Work out the finished part from the listing and answer in its coordinate system (mm). Round coordinates to 2 decimals unless told otherwise and drop trailing zeros. Loops run counter-clockwise (first coordinate to the right, second up) from the corner with the lowest first, then second, coordinate; pieces in that order, holes last. Notation, with made-up numbers: (-1.5, 32.25) - (48.5, 32.25) arc R17 ccw to (48.5, 55.25) - close; hole circle Ø7 at (55.5, 14.5). An arc over 180 degrees is marked (long way). Answer as CSV lines item,"result". Start each with the question number.
Q1. Straight lines are drawn through the part: L1, parallel to Y at x = 168.5, z = -34.5; L2, parallel to Y at x = -163, z = -490.5. For each, find the intervals that lie inside material, in ascending order. Write a range as [from, to].
Q2. Each of these flat-tipped pins is pushed along its axis until it touches: pin 1 Ø1.5 at (x, z) = (-8.5, -291) entering from -Y; pin 2 Ø4 at (x, y) = (173, -57.5) entering from -Z; pin 3 Ø4 at (x, y) = (180, -59) entering from +Z. Where does it stop, or does it pass through?
Q3. Section A-A on x = -110.5 is taken. Write down the section's boundary in (y, z).
Q4. Section B-B on z = -164 is taken. Write down the section's boundary in (x, y).
```python
from build123d import *

# Parameters (mm, degrees)
F0_W        = 457.2
F0_H        = 1828.8
F1_DEPTH    = 50.8
F2_W        = 25.4
F2_H        = 254
F3_DEPTH    = 25.4
F4_T1_DEPTH = 361.4104165052
F5_W        = 12.7
F5_H        = 57.15
F6_DEPTH    = 417.2741922717


# Not quite as in the source:
# - a fillet or chamfer that OpenCascade refuses, or shapes differently, is made with other operations: its cross-section is extruded or revolved along the edge and cut away or added


with BuildPart() as f1:
    # F0 (on Front) → F1 (new body)
    with BuildSketch(Plane.XZ):
        Rectangle(F0_W, F0_H)
    extrude(amount=F1_DEPTH)

    # F2 (on face) → F3 (join)
    with BuildSketch(Plane.XZ.offset(50.8)):
        with Locations((175.9731922717, 0)):
            Rectangle(F2_W, F2_H)
    extrude(amount=F3_DEPTH)

    # F4: fillet of radius 101.6 on 2 edges, made by hand

    # F4_s2 → F4_t1 (cut)
    with BuildSketch(Plane.YZ.offset(-4.7320159809)):
        with BuildLine():
            ThreePointArc((-50.8, 127), (-69.6380976241, 95.7189411832), (-76.2, 59.797916699))
            Line((-76.2, 59.797916699), (-76.2, 127))
            Line((-76.2, 127), (-50.8, 127))
        make_face()
        with BuildLine():
            ThreePointArc((-50.8, -127), (-69.6380976241, -95.7189411832), (-76.2, -59.797916699))
            Line((-76.2, -59.797916699), (-76.2, -127))
            Line((-76.2, -127), (-50.8, -127))
        make_face()
    extrude(amount=F4_T1_DEPTH, mode=Mode.SUBTRACT)

    # F5 (on face) → F6 (cut, through all)
    with BuildSketch(Plane.YZ.offset(188.6731922717)):
        with Locations((-57.15, -28.575)):
            Rectangle(F5_W, F5_H)
        with Locations((-57.15, 28.575)):
            Rectangle(F5_W, F5_H)
    extrude(amount=-F6_DEPTH, mode=Mode.SUBTRACT)


solid = f1.part
```
Findings:
1,L1,"y = [-76.2, -63.5], [-50.8, 0]"
1,L2,"y = [-50.8, 0]"
2,pin 1,"stops at y = -50.8"
2,pin 2,"stops at z = -121.26"
2,pin 3,"stops at z = 119.24"
3,outline,"(-50.8, -914.4) - (0, -914.4) - (0, 914.4) - (-50.8, 914.4) - close"
4,outline,"(-228.6, -50.8) - (228.6, -50.8) - (228.6, 0) - (-228.6, 0) - close"
